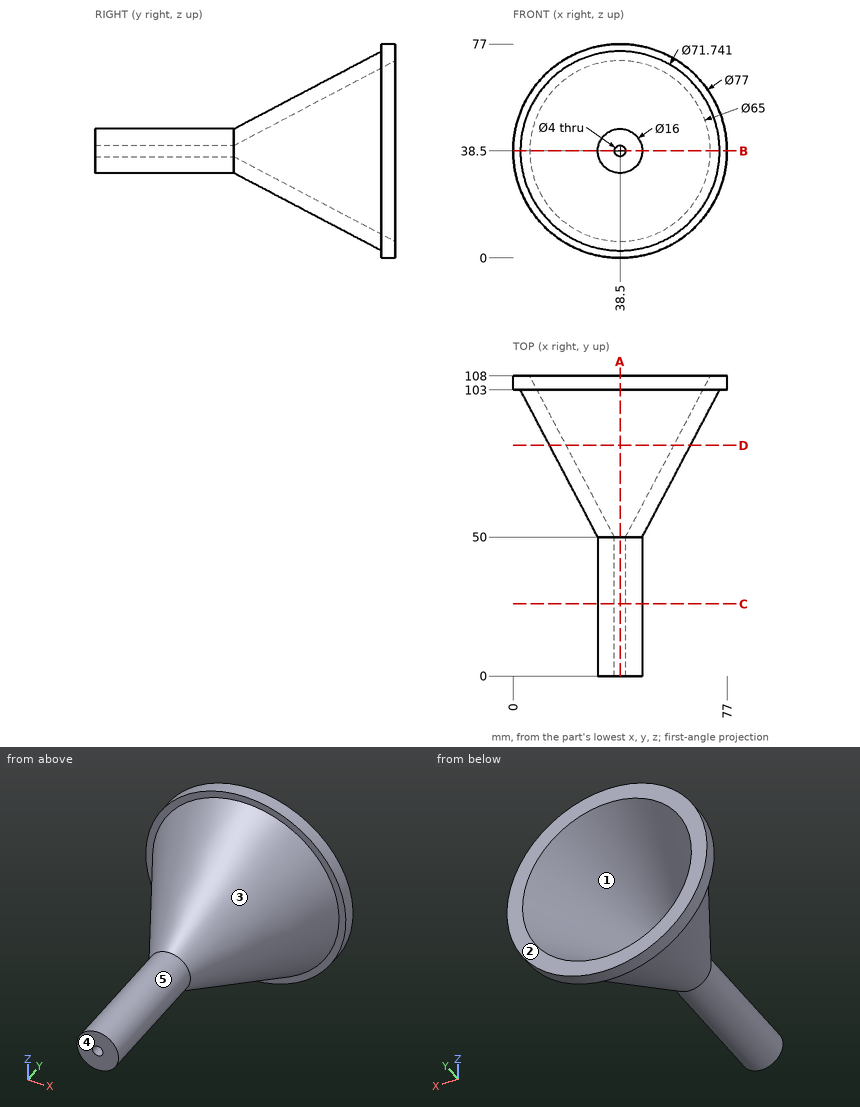
The drawing under review shows one solid part. Ordinate dimensions are in mm from its lowest x, y, z. A direction names the side the tool comes from. Coordinates: 2 decimals unless noted, no trailing zeros. Order: outer loops, then holes, each group sorted by start corner. A loop starts at its lowest first (then second) coordinate and runs counter-clockwise, first axis right, second up. Notation, with made-up numbers: (-22.5, -35.5) -> (18.5, -35.5) arc R23 cw to (18.5, -7.5) -> close; hole circle Ø10 at (-20, 30). An arc over 180 degrees is marked (long way). Answer in a Markdown table with one row per item. Add a question column.
Item 1: Clearance check with flat-ended pins moving along their axes: pin 1 (3 mm diameter, centred on x = 16.5, z = 39, fed in from -Y); pin 2 (12 mm diameter, centred on x = 45, z = 57, fed in from -Y) (1 decimal); pin 3 (10 mm diameter, centred on x = 48.5, z = 60.5, fed in from +Y). State where each tip first meets the part, or that it passes through.
Item 2: We need section A-A on x = 38.5. Write out the cut boundary in (y, z), plus the area to 3 significant figures.
Item 3: Mouldability with a two-part tool opening along X and no side actions: class the marked faces 1, 2 and 3 as +X half, -X half, draft (parallel to the pull), parting line (faces both ways), or undercut.
Item 4: Machinability: for the marked faces 4 and 5, which of the approach directions +Z, -Z, +X, -X, +Y, -Y give a long, thin tool a straight path to every point of the face, cutting with its end or side? Answer none if there is none.
Item 5: We need section D-D on y = 83. Write out the cut boundary in (x, z).
Item 6: We need section B-B on z = 38.5. Write out the cut boundary in (x, y).
Item 7: We need section C-C on y = 26. Write out the cut boundary in (x, z).
Item 8: To check wall thickness, follow probe 1 along X at (y, z) = (12.5, 38.5); probe 2 along Y at (x, z) = (65, 14). State the ranges of each line that lie inside material, in increasing order.
Final values:
| question | item | result |
|---|---|---|
| 1 | pin 1 | stops at y = 73.78 |
| 1 | pin 2 | stops at y = 60.7 |
| 1 | pin 3 | stops at y = 101.66 |
| 2 | outline | (0, 30.5) -> (50, 30.5) -> (103, 2.63) -> (103, 0) -> (108, 0) -> (108, 6) -> (50, 36.5) -> (0, 36.5) -> close; (0, 40.5) -> (50, 40.5) -> (108, 71) -> (108, 77) -> (103, 77) -> (103, 74.37) -> (50, 46.5) -> (0, 46.5) -> close |
| 2 | area | 1,310 mm2 |
| 3 | face 1 | undercut |
| 3 | face 2 | draft |
| 3 | face 3 | parting line |
| 4 | face 4 | +Z, -Z, +X, -X, -Y |
| 4 | face 5 | -Y |
| 5 | outline | circle Ø50.71 at (38.5, 38.5); hole circle Ø38.71 at (38.5, 38.5) |
| 6 | outline | (0, 103) -> (2.63, 103) -> (30.5, 50) -> (30.5, 0) -> (36.5, 0) -> (36.5, 50) -> (6, 108) -> (0, 108) -> close; (40.5, 0) -> (46.5, 0) -> (46.5, 50) -> (74.37, 103) -> (77, 103) -> (77, 108) -> (71, 108) -> (40.5, 50) -> close |
| 7 | outline | circle Ø16 at (38.5, 38.5); hole circle Ø4 at (38.5, 38.5) |
| 8 | probe 1 | x = 30.5 to 36.5, 40.5 to 46.5 |
| 8 | probe 2 | y = 103 to 108 |
